Build history of the part. All positions in model axes, mm. Round coordinates to 2 decimals unless told otherwise and drop trailing zeros. Loops run counter-clockwise (first coordinate to the right, second up) from the corner with the lowest first, then second, coordinate; pieces in that order, holes last.
from build123d import *

# Parameters (mm, degrees)
SKETCH1_R            = 9.525
EXTRUDE1_DEPTH       = 19.05
CHAMFER1_SIZE        = 0.4064
TRUNCATED_DEPTH      = 20.05
TRUNCATED_DEPTH_BACK = 20.05


with BuildPart() as part:
    # Sketch1 → Extrude1 (new body, symmetric)
    with BuildSketch(Plane.XY):
        Circle(SKETCH1_R)
    extrude(amount=EXTRUDE1_DEPTH, both=True)

    # Chamfer1
    chamfer1_edges = [part.edges().sort_by_distance(p)[0] for p in [
        (-9.525, 0, -19.05),
        (-9.525, 0, 19.05),
    ]]
    chamfer(chamfer1_edges, length=CHAMFER1_SIZE)

    # Sketch2 → Truncated (cut, two sides)
    with BuildSketch(Plane.XY) as truncated_sk:
        with BuildLine():
            Line((-8.980256121, -3.175), (8.980256121, -3.175))
            ThreePointArc((8.980256121, -3.175), (0, -9.525), (-8.980256121, -3.175))
        make_face()
    extrude(amount=TRUNCATED_DEPTH, mode=Mode.SUBTRACT)
    extrude(truncated_sk.sketch, amount=-TRUNCATED_DEPTH_BACK, mode=Mode.SUBTRACT)


solid = part.part
(1) Slice it at A-A on z = 9. List the corners of the cut face in (x, y) (3 decimals).
Responses:
outline: (-8.98, -3.175) - (8.98, -3.175) arc R9.525 ccw (long way) to start
(2) Probe line 1 (X direction, y = 2.75, z = -14.5); line 2 (Y direction, x = -6.5, z = 1) (3 decimals); line 3 (Y direction, x = 3.5, z = 8) (3 decimals). List the from-to ranges inside material, lowest first.
Responses:
line 1: x = -9.12 to 9.12
line 2: y = -3.175 to 6.962
line 3: y = -3.175 to 8.859
(3) Pin check, flat tips, straight feed: P1, Ø1.5, axis at x = -3.5, z = 0.5, coming from the +Y side; P2, Ø3, axis at x = -6, z = 6, coming from the +Y side (3 decimals); P3, Ø5, axis at y = 3, z = -12, coming from the -X side. Stop position of each tip, or through.
Responses:
P1: stops at y = 9.12
P2: stops at y = 8.395
P3: stops at x = -9.51
